```python
from build123d import *

# Parameters (mm, degrees)
SKETCH1_W           = 76.2
SKETCH1_H           = 76.2
BOSS_EXTRUDE1_DEPTH = 6.35
SKETCH2_W           = 6.604
SKETCH2_H           = 48.006
CUT_EXTRUDE1_DEPTH  = 55.254423783
SKETCH3_R           = 3.175
CUT_EXTRUDE3_DEPTH  = 55.254423783


with BuildPart() as part:
    # Sketch1 → Boss-Extrude1 (new body)
    with BuildSketch(Plane(origin=(0, 0, 0), x_dir=(1, 0, 0), z_dir=(0, 1, 0))):
        Rectangle(SKETCH1_W, SKETCH1_H)
    extrude(amount=BOSS_EXTRUDE1_DEPTH)

    # Sketch2 → Cut-Extrude1 (cut, through all)
    with BuildSketch(Plane(origin=(0, 0, 0), x_dir=(1, 0, 0), z_dir=(0, 1, 0))):
        with Locations((16.002, 0)):
            Rectangle(SKETCH2_W, SKETCH2_H)
        with Locations((-16.002, 0)):
            Rectangle(SKETCH2_W, SKETCH2_H)
    extrude(amount=CUT_EXTRUDE1_DEPTH, mode=Mode.SUBTRACT)

    # Sketch3 → Cut-Extrude3 (cut, through all)
    with BuildSketch(Plane(origin=(0, 0, 0), x_dir=(1, 0, 0), z_dir=(0, 1, 0))):
        with Locations(Location((-16.002, 30.48, 0), (0, 0, 270))):
            Circle(SKETCH3_R)
        with Locations(Location((-16.002, -30.48, 0), (0, 0, 90))):
            Circle(SKETCH3_R)
        with Locations(Location((16.002, -30.48, 0), (0, 0, 270))):
            Circle(SKETCH3_R)
        with Locations(Location((16.002, 30.48, 0), (0, 0, 90))):
            Circle(SKETCH3_R)
    extrude(amount=CUT_EXTRUDE3_DEPTH, mode=Mode.SUBTRACT)


solid = part.part
```
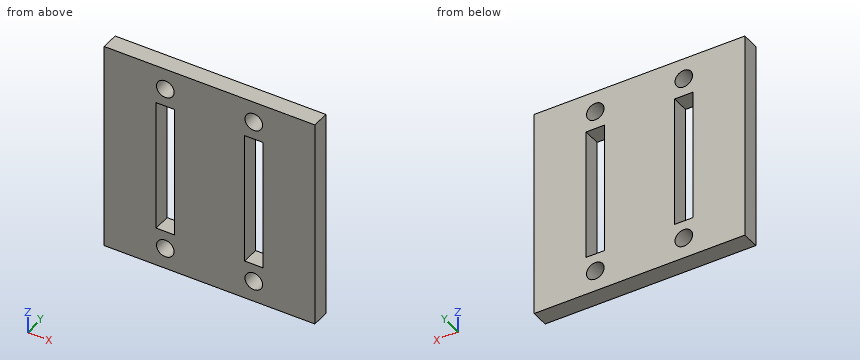
For this review, take the finished solid that the model builds, in its own axes (mm). Round coordinates to 2 decimals unless told otherwise and drop trailing zeros. Order: outer loops, then holes, each group sorted by start corner. A loop starts at its lowest first (then second) coordinate and runs counter-clockwise, first axis right, second up. Notation, with made-up numbers: (55.25, 55) -> (73.25, 55) arc R24 cw to (73.25, 84) -> close; hole circle Ø8 at (44.25, -15.5). An arc over 180 degrees is marked (long way). Use a Markdown table: item, result.
Item 1: For line 1 along X through (y, z) = (3.25, 30.48); line 2 along X through (y, z) = (4.5, 6.5); line 3 along Z through (x, y) = (15, 3.5), list the stretches that pass through material, from the lowest coordinate up. Write a range as [from, to].
Resolved:
| item | result |
|---|---|
| line 1 | x = [-38.1, -19.18], [-12.83, 12.83], [19.18, 38.1] |
| line 2 | x = [-38.1, -19.3], [-12.7, 12.7], [19.3, 38.1] |
| line 3 | z = [-38.1, -33.49], [-27.47, -24], [24, 27.47], [33.49, 38.1] |
Item 2: Take a section at B-B (y = 4.5). State the section outline as (x, z) points (3 decimals).
Resolved:
| item | result |
|---|---|
| outline | (-38.1, -38.1) -> (38.1, -38.1) -> (38.1, 38.1) -> (-38.1, 38.1) -> close; hole (-19.304, -24.003) -> (-12.7, -24.003) -> (-12.7, 24.003) -> (-19.304, 24.003) -> close; hole circle Ø6.35 at (-16.002, -30.48); hole circle Ø6.35 at (-16.002, 30.48); hole (12.7, -24.003) -> (19.304, -24.003) -> (19.304, 24.003) -> (12.7, 24.003) -> close; hole circle Ø6.35 at (16.002, -30.48); hole circle Ø6.35 at (16.002, 30.48) |
Item 3: Take a section at C-C (z = -30.48). State the section outline as (x, y) points, plus the area to 3 significant figures.
Resolved:
| item | result |
|---|---|
| outline | (-38.1, 0) -> (-19.18, 0) -> (-19.18, 6.35) -> (-38.1, 6.35) -> close; (-12.83, 0) -> (12.83, 0) -> (12.83, 6.35) -> (-12.83, 6.35) -> close; (19.18, 0) -> (38.1, 0) -> (38.1, 6.35) -> (19.18, 6.35) -> close |
| area | 403 mm² |
Item 4: Take a section at A-A (z = 13.5). State the section outline as (x, y) points.
Resolved:
| item | result |
|---|---|
| outline | (-38.1, 0) -> (-19.3, 0) -> (-19.3, 6.35) -> (-38.1, 6.35) -> close; (-12.7, 0) -> (12.7, 0) -> (12.7, 6.35) -> (-12.7, 6.35) -> close; (19.3, 0) -> (38.1, 0) -> (38.1, 6.35) -> (19.3, 6.35) -> close |
